Input: part model. Units: mm. Frame: model coordinates. Face numbers are marked on the shaded views. A direction names the side the tool comes from. Round coordinates to 2 decimals unless told otherwise and drop trailing zeros. Loops run counter-clockwise (first coordinate to the right, second up) from the corner with the lowest first, then second, coordinate; pieces in that order, holes last.
1) Access query for the marked faces 4, 5 and 6. Directions: +Z, -Z, +X, -X, +Y, -Y. A direction counts if a zero-diameter tool reaches every point of the face in a straight line with its end or side. Return the directions, or none.
2) Section B-B, the plane z = -6.75. Return loops of the section in (x, y), and give its area (4 significant figures).
3) Section D-D, the plane y = -1.75. Return loops of the section in (x, z), and give its area (3 significant figures).
4) Draft query along Z for the marked faces 1, 2 and 3. Return one class per face: pulls with the +Z half, pulls with the -Z half, needs draft (parallel to the pull), parting line crosses it, or undercut.
5) Section A-A, the plane y = 3. Return loops of the section in (x, z), and give its area (4 significant figures).
6) First-contact query: pin 1 (6 mm diameter, centred on x = -12, z = -3.5, fed in from -Y); pin 2 (5 mm diameter, centred on x = -0.5, z = 0, fed in from +Y); pin 3 (3.5 mm diameter, centred on x = 4, y = 3.5, fed in from +Z). Flat tips, straight axial feed; report the tip coordinate or a pass-through.
7) Section C-C, the plane x = -1. Return loops of the section in (y, z), and give its area (3 significant figures).
8) Ray query, line 1 along Z through (x, y) = (-6, 3); line 2 along X through (y, z) = (1.25, -6); line 3 along Y through (x, z) = (-16, -6.5). Return the intervals inside material, ascending.
from build123d import *

# Parameters (mm, degrees)
SKETCH1_W           = 35.5
SKETCH1_H           = 17.68
BOSS_EXTRUDE1_DEPTH = 1.6
SKETCH2_W           = 34.9
SKETCH2_H           = 2.5
BOSS_EXTRUDE2_DEPTH = 3
SKETCH3_W           = 5.6
SKETCH3_H           = 8
BOSS_EXTRUDE3_DEPTH = 3


with BuildPart() as part:
    # Sketch1 → Boss-Extrude1 (new body)
    with BuildSketch(Plane(origin=(0, 0, 0), x_dir=(1, 0, 0), z_dir=(0, 1, 0))):
        Rectangle(SKETCH1_W, SKETCH1_H)
    extrude(amount=BOSS_EXTRUDE1_DEPTH)

    # Sketch2 → Boss-Extrude2 (add)
    with BuildSketch(Plane(origin=(0, 1.6, 0), x_dir=(1, 0, 0), z_dir=(0, 1, 0))):
        with Locations((0, 7.39)):
            Rectangle(SKETCH2_W, SKETCH2_H)
        with Locations((0, -7.39)):
            Rectangle(SKETCH2_W, SKETCH2_H)
    extrude(amount=BOSS_EXTRUDE2_DEPTH)

    # Sketch3 → Boss-Extrude3 (add)
    with BuildSketch(Plane.XZ):
        with Locations((15.95, 0)):
            Rectangle(SKETCH3_W, SKETCH3_H)
    extrude(amount=BOSS_EXTRUDE3_DEPTH)


solid = part.part
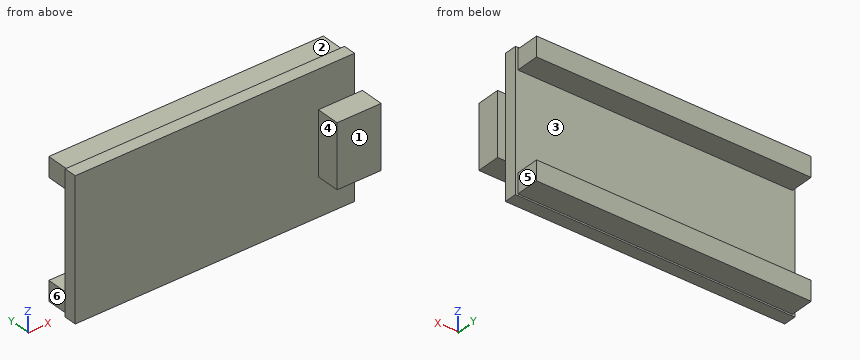
Final values:
1. face 4: +Z, -Z, -X, -Y
1. face 5: +Z, -Z, +X, +Y
1. face 6: +Z, -Z, -X, +Y
2. outline: (-17.75, 0) - (17.75, 0) - (17.75, 1.6) - (17.45, 1.6) - (17.45, 4.6) - (-17.45, 4.6) - (-17.45, 1.6) - (-17.75, 1.6) - close
2. area: 161.5 mm2
3. outline: (13.15, -4) - (18.75, -4) - (18.75, 4) - (13.15, 4) - close
3. area: 44.8 mm2
4. face 1: needs draft
4. face 2: pulls with the +Z half
4. face 3: undercut
5. outline: (-17.45, -8.64) - (17.45, -8.64) - (17.45, -6.14) - (-17.45, -6.14) - close; (-17.45, 6.14) - (17.45, 6.14) - (17.45, 8.64) - (-17.45, 8.64) - close
5. area: 174.5 mm2
6. pin 1: stops at y = 0
6. pin 2: stops at y = 1.6
6. pin 3: stops at z = 8.64
7. outline: (0, -8.84) - (1.6, -8.84) - (1.6, -8.64) - (4.6, -8.64) - (4.6, -6.14) - (1.6, -6.14) - (1.6, 6.14) - (4.6, 6.14) - (4.6, 8.64) - (1.6, 8.64) - (1.6, 8.84) - (0, 8.84) - close
7. area: 43.3 mm2
8. line 1: z = -8.64 to -6.14, 6.14 to 8.64
8. line 2: x = -17.75 to 17.75
8. line 3: y = 0 to 4.6
